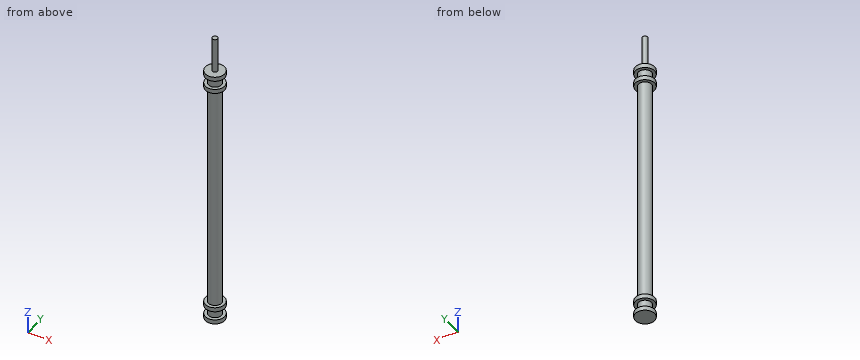
from build123d import *

# Parameters (mm, degrees)
SKETCH1_R           = 3.725
BOSS_EXTRUDE1_DEPTH = 132
SKETCH3_R           = 5.5
BOSS_EXTRUDE3_DEPTH = 2.5
SKETCH4_R           = 3.725
BOSS_EXTRUDE4_DEPTH = 5
SKETCH5_R           = 5.5
BOSS_EXTRUDE5_DEPTH = 2.5
SKETCH6_R           = 1.5
BOSS_EXTRUDE6_DEPTH = 20


with BuildPart() as part:
    # Sketch1 → Boss-Extrude1 (new body)
    with BuildSketch(Plane.XY):
        Circle(SKETCH1_R)
    extrude(amount=BOSS_EXTRUDE1_DEPTH)

    # Sketch3 → Boss-Extrude3 (add)
    with BuildSketch(Plane.XY.offset(132)):
        Circle(SKETCH3_R)
    boss_extrude3 = extrude(amount=BOSS_EXTRUDE3_DEPTH)

    # Sketch4 → Boss-Extrude4 (add)
    with BuildSketch(Plane.XY.offset(134.5)):
        Circle(SKETCH4_R)
    boss_extrude4 = extrude(amount=BOSS_EXTRUDE4_DEPTH)

    # Sketch5 → Boss-Extrude5 (add)
    with BuildSketch(Plane.XY.offset(139.5)):
        Circle(SKETCH5_R)
    boss_extrude5 = extrude(amount=BOSS_EXTRUDE5_DEPTH)

    # Mirror2: Boss-Extrude3, Boss-Extrude4, Boss-Extrude5 across plane
    add(boss_extrude3.mirror(Plane.XY.offset(66)))
    add(boss_extrude4.mirror(Plane.XY.offset(66)))
    add(boss_extrude5.mirror(Plane.XY.offset(66)))

    # Sketch6 → Boss-Extrude6 (add)
    with BuildSketch(Plane.XY.offset(142)):
        Circle(SKETCH6_R)
    extrude(amount=BOSS_EXTRUDE6_DEPTH)


solid = part.part
Build history of the part. All positions in model axes, mm. Give positions to 0.01 mm unless a question says otherwise; leave off trailing zeros. Loops run counter-clockwise (first coordinate to the right, second up) from the corner with the lowest first, then second, coordinate; pieces in that order, holes last. Notation, with made-up numbers: (50, 22) -> (86, 22) arc R20 cw to (86, 39) -> close; hole circle Ø8 at (-30.5, -11.5). An arc over 180 degrees is marked (long way). Answer in a Markdown table with one row per item.
Item 1: Flat gauge pins, fed straight in: P1, Ø3, axis at y = -1, z = 30, coming from the +X side (3 decimals); P2, Ø1.5, axis at x = 0.5, z = 137.5, coming from the -Y side (3 decimals); P3, Ø6, axis at y = -4, z = 55.5, coming from the +X side. Where does each tip first touch, or does it go through?
Findings below:
| item | result |
|---|---|
| P1 | stops at x = 3.725 |
| P2 | stops at y = -3.725 |
| P3 | stops at x = 3.59 |
Item 2: Slice it at C-C on z = 31. Write the cut outline in (x, y) (3 decimals), plus the area to 3 significant figures.
Findings below:
| item | result |
|---|---|
| outline | circle Ø7.45 at (0, 0) |
| area | 43.6 mm² |
Item 3: Probe line 1 along Z through (x, y) = (5.25, -1.5); line 2 along Y through (x, z) = (0.5, 23); line 3 along X through (y, z) = (-0.25, 81.5). List the from-to ranges inside material, lowest first. Write a range as [from, to].
Findings below:
| item | result |
|---|---|
| line 1 | z = [-10, -7.5], [-2.5, 0], [132, 134.5], [139.5, 142] |
| line 2 | y = [-3.69, 3.69] |
| line 3 | x = [-3.72, 3.72] |
